The figure shows three views and two pictorial views of one solid part (mm, origin at its lowest corner). Answer the questions. A direction names the side the tool comes from. Coordinates: 2 decimals unless noted, no trailing zeros. Order: outer loops, then holes, each group sorted by start corner. A loop starts at its lowest first (then second) coordinate and runs counter-clockwise, first axis right, second up. Notation, with made-up numbers: (42, -2) -> (51, -2) arc R10 ccw to (51, 2) -> close; hole circle Ø8 at (7, 14.25). An arc over 180 degrees is marked (long way). Return JSON: item names as keys, results as strings. Group by question number.
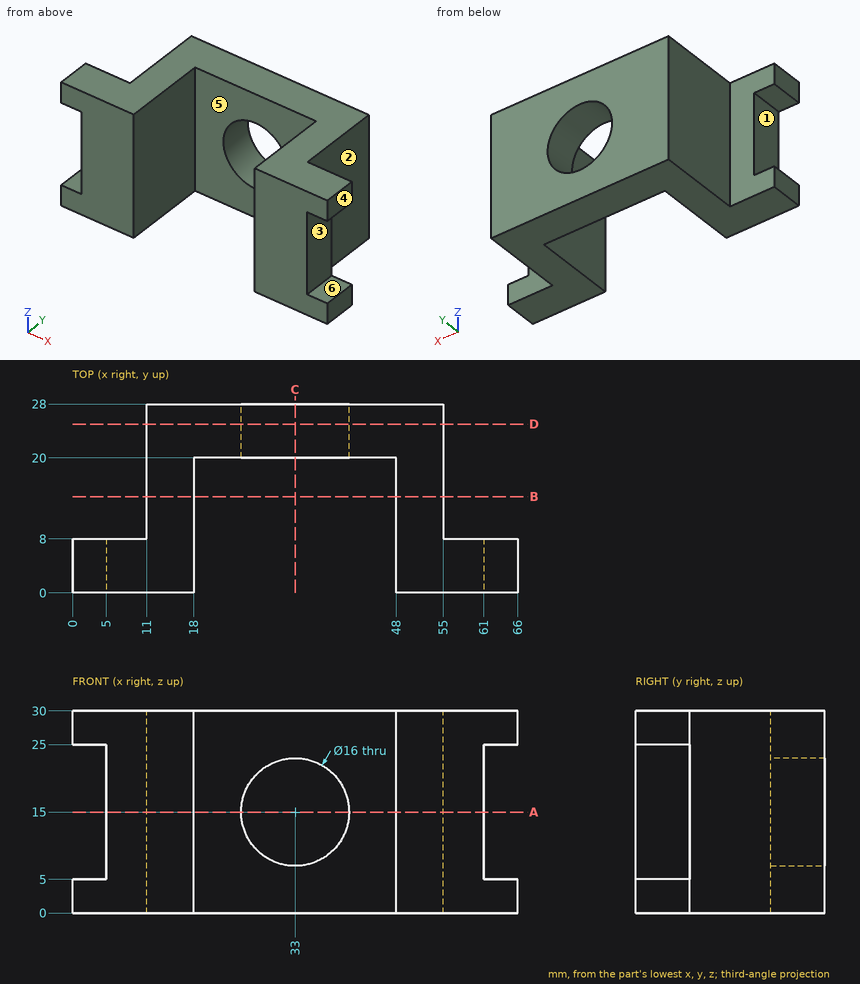
1. For a pull along X with two mould halves and no side action, classify the marked faces 4, 5 and 6 as released by +X, released by -X, zero draft, split by the parting line, or undercut.
2. Straight lines are drawn through the part: L1, parallel to X at y = 7, z = 27.75; L2, parallel to X at y = 24.75, z = 15; L3, parallel to Y at x = 10.5, z = 22.25. For each, find the intervals that lie inside material, in ascending order.
3. Find section B-B on y = 14.25. Determine the outline of the cut face in (x, z), and give its area (3 significant figures).
4. Find section D-D on y = 25. Determine the outline of the cut face in (x, z), and give its area (3 significant figures).
5. Find section C-C on x = 33. Determine the outline of the cut face in (y, z).
6. Given pin 1 (9 mm diameter, centred on y = 5.5, z = 13, fed in from -X); pin 2 (2 mm diameter, centred on y = 12, z = 8, fed in from +X); pin 3 (12 mm diameter, centred on x = 3, z = 9, fed in from +Y), each flat-ended and moving along its own axis, determine where each tip first touches the part or whether it passes through.
7. Find section A-A on z = 15. Determine the outline of the cut face in (x, y).
8. Which of the six approach directions +Z, -Z, +X, -X, +Y, -Y give full straight-line access (tool end or side, diameter ignored) to the marked faces 1, 2 and 3?
Result:
{
 "1": {"face 4": "released by +X", "face 5": "undercut", "face 6": "zero draft"},
 "2": {"L1": "0 to 18, 48 to 66", "L2": "11 to 25, 41 to 55", "L3": "0 to 8"},
 "3": {"outline": "(11, 0) -> (18, 0) -> (18, 30) -> (11, 30) -> close; (48, 0) -> (55, 0) -> (55, 30) -> (48, 30) -> close", "area": "420 mm^2"},
 "4": {"outline": "(11, 0) -> (55, 0) -> (55, 30) -> (11, 30) -> close; hole circle Ø16 at (33, 15)", "area": "1,120 mm^2"},
 "5": {"outline": "(20, 0) -> (28, 0) -> (28, 7) -> (20, 7) -> close; (20, 23) -> (28, 23) -> (28, 30) -> (20, 30) -> close"},
 "6": {"pin 1": "x = 5", "pin 2": "x = 55", "pin 3": "y = 8"},
 "7": {"outline": "(5, 0) -> (18, 0) -> (18, 20) -> (25, 20) -> (25, 28) -> (11, 28) -> (11, 8) -> (5, 8) -> close; (41, 20) -> (48, 20) -> (48, 0) -> (61, 0) -> (61, 8) -> (55, 8) -> (55, 28) -> (41, 28) -> close"},
 "8": {"face 1": "-X, +Y, -Y", "face 2": "+Z, -Z, +X, +Y", "face 3": "+X, +Y, -Y"}
}
